Can you work these out from the model? Positions are in its coordinate system, mm. Face numbers are marked on the shaded views. A direction names the side the tool comes from. Coordinates: 2 decimals unless noted, no trailing zeros. Write each loop counter-clockwise with the first axis right and the second up, starting at its lowest first coordinate (ties: lowest second). Pieces come first, ordered by that corner, then holes. Notation, with made-up numbers: (53.25, 9) - (86.25, 9) arc R20 cw to (86.25, 45) - close; hole circle Ø2 at (10, 45). An arc over 180 degrees is marked (long way). One line per question, with ' | ' between items. Start each with the question number.
from build123d import *

# Parameters (mm, degrees)
SKETCH1_R               = 11
SKETCH1_R_2             = 8.25
BOSS_EXTRUDE1_DEPTH     = 20
BOSS_EXTRUDE2_START     = 10.5
SKETCH2_W               = 22
SKETCH2_H               = 40
BOSS_EXTRUDE2_DEPTH     = 5
FILLET1_R               = 10
CUT_EXTRUDE1_DEPTH      = 32.356817441
CUT_EXTRUDE1_DEPTH_BACK = 32.356817441
SKETCH3_R               = 2
CUT_EXTRUDE2_DEPTH      = 3


with BuildPart() as part:
    # Sketch1 → Boss-Extrude1 (new body)
    with BuildSketch(Plane.XY):
        Circle(SKETCH1_R)
        Circle(SKETCH1_R_2, mode=Mode.SUBTRACT)
    extrude(amount=BOSS_EXTRUDE1_DEPTH)

    # Sketch2 → Boss-Extrude2 (add)
    with BuildSketch(Plane(origin=(0, 0, 0), x_dir=(1, 0, 0), z_dir=(0, 1, 0)).offset(BOSS_EXTRUDE2_START)):
        Rectangle(SKETCH2_W, SKETCH2_H)
    extrude(amount=BOSS_EXTRUDE2_DEPTH)

    # Fillet1
    # the kernel refuses this fillet: 10 mm, written as the material it adds along each edge
    with BuildSketch(Plane(origin=(-3.278719262, 10.5, 20), x_dir=(-0.7068612183411899, -0.7073522587828561, 0), z_dir=(0, 0, -1))) as fillet1_piece_1:
        with BuildLine():
            CenterArc((14.864288654, 8.855683881), FILLET1_R, 199.840435799, 42.481112875)
            Line((5.45787391, 5.461665371), (5.269745615, 5.393785))
            ThreePointArc((5.269745615, 5.393785), (2.587466503, 2.872204929), (-0.141470452, 0.141372244))
            Line((-0.141470452, 0.141372244), (0.092901804, -0.177113678))
            ThreePointArc((0.092901804, -0.177113678), (5.109599225, 1.058747731), (10.126296646, -0.177113678))
            Line((10.126296646, -0.177113678), (10.21919845, 0))
        make_face()
    extrude(amount=20)
    with BuildSketch(Plane(origin=(3.278719262, 10.5, 20), x_dir=(0.7068612183411898, -0.7073522587828562, 0), z_dir=(0, 0, -1))) as fillet1_piece_2:
        with BuildLine():
            CenterArc((14.864288654, -8.855683881), FILLET1_R, 117.678451325, 42.481112875)
            Line((5.45787391, -5.461665371), (5.269745615, -5.393785))
            ThreePointArc((5.269745615, -5.393785), (2.587466503, -2.872204929), (-0.141470452, -0.141372244))
            Line((-0.141470452, -0.141372244), (0.092901804, 0.177113678))
            ThreePointArc((0.092901804, 0.177113678), (5.109599225, -1.058747731), (10.126296646, 0.177113678))
            Line((10.126296646, 0.177113678), (10.21919845, 0))
        make_face()
    extrude(amount=20)

    # Sketch3 → Cut-Extrude1 (cut, two sides: drawn at the far end of the back side and taken through both)
    with BuildSketch(Plane.XZ.offset(-10.5).offset(-CUT_EXTRUDE1_DEPTH_BACK)):
        with Locations(Location((0, -9, 0), (0, 0, 270))):
            Circle(SKETCH3_R)
        with BuildLine():
            Line((-11, -9), (-17.508128505, -13.92083612))
            Line((-17.508128505, -13.92083612), (-14.254064253, -21.523754309))
            Line((-14.254064253, -21.523754309), (21.256045922, -20))
            Line((21.256045922, -20), (18.95789911, -14.630523296))
            Line((18.95789911, -14.630523296), (11, -9))
            ThreePointArc((11, -9), (0, -20), (-11, -9))
        make_face()
    extrude(amount=CUT_EXTRUDE1_DEPTH + CUT_EXTRUDE1_DEPTH_BACK, mode=Mode.SUBTRACT)

    # Sketch4 → Cut-Extrude2 (cut)
    with BuildSketch(Plane.XZ.offset(-10.5)):
        Polygon((3.5, -6.979274058), (0, -4.958548116), (-3.5, -6.979274058), (-3.5, -11.020725942), (0, -13.041451884), (3.5, -11.020725942), align=None)
    extrude(amount=-CUT_EXTRUDE2_DEPTH, mode=Mode.SUBTRACT)


solid = part.part
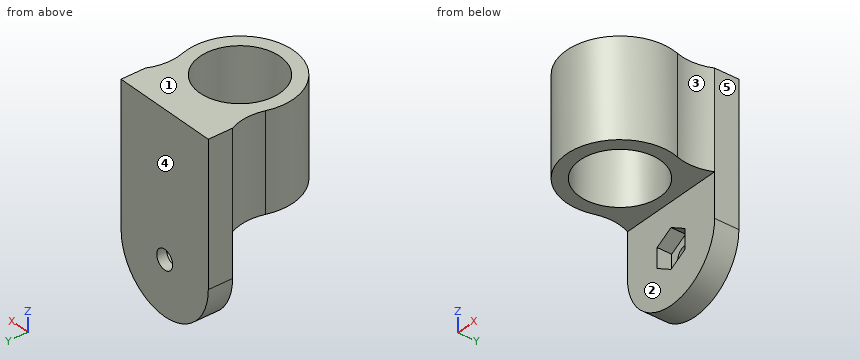
(1) If I drill on probe 1 along X at (y, z) = (15.05, -9); probe 2 along Y at (x, z) = (0, 14); probe 3 along Y at (x, z) = (7.75, -5.5), over which ranges is the centre line in solid material (lowest first)?
(2) Which directions (+Z, -Z, +X, -X, +Y, -Y) give clear straight access to the entire face, cutting with the end or side of a thin tool? Please do the marked faces 1 and 2.
(3) I'm going to push flat-ended pins straight in: pin 1 (10 mm diameter, centred on x = 2, z = -15, fed in from -Y); pin 2 (2 mm diameter, centred on x = -6, y = 7.5, fed in from -Z); pin 3 (3.5 mm diameter, centred on x = -1, z = -9.5, fed in from -Y); pin 4 (3 mm diameter, centred on x = -2, y = -5.5, fed in from +Z). Where does each tip first touch, or does it pass through?
(4) If we section it at D-D on z = 15: List the corners of the cut face in (x, y) for me.
(5) If we section it at C-C on z = -9.5: List the corners of the cut face in (x, y) for me, plus the area to 3 significant figures.
(6) If we section it at B-B on x = -6.25: List the corners of the cut face in (y, z) for me, plus the area to 3 significant figures.
(7) If we mould it in two halves opening along Y, with no side actions, what happens to the marked faces 3, 4 and 5? For each: +Y half, -Y half, draft (parallel to the pull), parting line (faces both ways), or undercut.
(8) If we section it at A-A on y = 0: List the corners of the cut face in (x, z) for me, plus the area to 3 significant figures.
Values:
1) probe 1: -11 to -2, 2 to 11 | probe 2: -11 to -8.25, 8.25 to 15.5 | probe 3: 10.5 to 15.5
2) face 1: +Z, +X, -X, +Y, -Y | face 2: -Z, +X, -X, -Y
3) pin 1: y = 10.5 | pin 2: z = 0 | pin 3: y = 13.5 | pin 4: through
4) outline: (-11, 10.5) arc R10 cw to (-10.5, 3.27) arc R11 ccw (long way) to (10.5, 3.27) arc R10 cw to (11, 10.5) - (11, 15.5) - (-11, 15.5) - close; hole circle Ø16.5 at (0, 0)
5) outline: (-10.99, 10.5) - (-3.5, 10.5) - (-3.5, 13.5) - (-1.94, 13.5) - (-1.94, 15.5) - (-10.99, 15.5) - close; (1.94, 13.5) - (3.5, 13.5) - (3.5, 10.5) - (10.99, 10.5) - (10.99, 15.5) - (1.94, 15.5) - close | area: 81.1 mm2
6) outline: (-9.05, 0) - (-5.39, 0) - (-5.39, 20) - (-9.05, 20) - close; (5.39, 0) - (10.5, 0) - (10.5, -18.05) - (15.5, -18.05) - (15.5, 20) - (5.39, 20) - close | area: 366 mm2
7) face 3: undercut | face 4: +Y half | face 5: draft
8) outline: (-11, 0) - (-8.25, 0) - (-8.25, 20) - (-11, 20) - close; (8.25, 0) - (11, 0) - (11, 20) - (8.25, 20) - close | area: 110 mm2
